For this review, take the finished solid that the model builds, in its own axes (mm). Face numbers are marked on the shaded views. Give positions to 0.01 mm unless a question says otherwise; leave off trailing zeros. Write each loop counter-clockwise with the first axis right and the second up, starting at its lowest first coordinate (ties: lowest second). Pieces come first, ordered by that corner, then holes. Notation, with made-up numbers: M 17.25,-8 L 54.25,-8 A13 ccw 54.25,8 Z; hole C 1,-13.5 d2. An arc over 180 degrees is marked long. Answer as a JSON object with one key per item and string values. Group by question number.
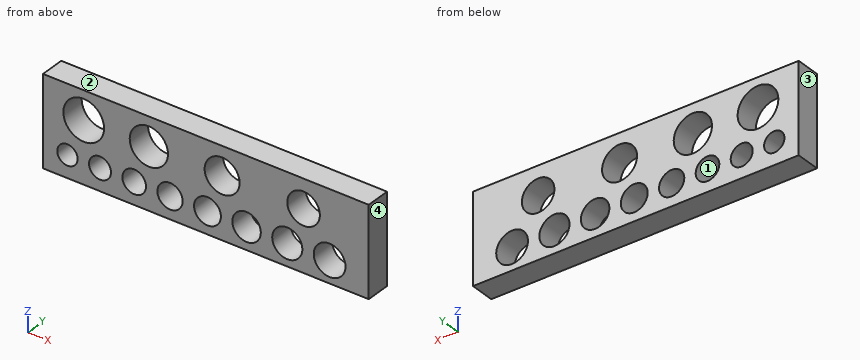
```python
from build123d import *

# Parameters (mm, degrees)
SKETCH1_W           = 40
SKETCH1_H           = 11
BOSS_EXTRUDE1_DEPTH = 3
SKETCH2_R           = 1.25
SKETCH2_R_2         = 1.35
SKETCH2_R_3         = 1.45
SKETCH2_R_4         = 1.55
SKETCH2_R_5         = 1.65
SKETCH2_R_6         = 1.75
SKETCH2_R_7         = 1.85
SKETCH2_R_8         = 1.95
SKETCH2_R_9         = 2.15
SKETCH2_R_10        = 2
SKETCH2_R_11        = 2.5
SKETCH2_R_12        = 2.35
CUT_EXTRUDE1_DEPTH  = 21.958291915


with BuildPart() as part:
    # Sketch1 → Boss-Extrude1 (new body)
    with BuildSketch(Plane(origin=(0, 0, 0), x_dir=(1, 0, 0), z_dir=(0, 1, 0))):
        Rectangle(SKETCH1_W, SKETCH1_H)
    extrude(amount=BOSS_EXTRUDE1_DEPTH)

    # Sketch2 → Cut-Extrude1 (cut, through all)
    with BuildSketch(Plane(origin=(0, 3, 0), x_dir=(1, 0, 0), z_dir=(0, 1, 0))):
        with Locations(Location((-17, 2.8, 0), (0, 0, 270))):
            Circle(SKETCH2_R)
        with Locations(Location((-13, 2.8, 0), (0, 0, 270))):
            Circle(SKETCH2_R_2)
        with Locations(Location((-8.8, 2.8, 0), (0, 0, 270))):
            Circle(SKETCH2_R_3)
        with Locations(Location((-4.4, 2.8, 0), (0, 0, 270))):
            Circle(SKETCH2_R_4)
        with Locations(Location((0.2, 2.8, 0), (0, 0, 270))):
            Circle(SKETCH2_R_5)
        with Locations(Location((5, 2.8, 0), (0, 0, 270))):
            Circle(SKETCH2_R_6)
        with Locations(Location((10, 2.8, 0), (0, 0, 270))):
            Circle(SKETCH2_R_7)
        with Locations(Location((15.2, 2.8, 0), (0, 0, 270))):
            Circle(SKETCH2_R_8)
        with Locations(Location((2, -2, 0), (0, 0, 270))):
            Circle(SKETCH2_R_9)
        with Locations(Location((12, -2, 0), (0, 0, 270))):
            Circle(SKETCH2_R_10)
        with Locations(Location((-15, -2, 0), (0, 0, 270))):
            Circle(SKETCH2_R_11)
        with Locations(Location((-7, -2, 0), (0, 0, 270))):
            Circle(SKETCH2_R_12)
    extrude(amount=-CUT_EXTRUDE1_DEPTH, mode=Mode.SUBTRACT)


solid = part.part
```
Item 1: Consider section B-B (x = 5). Give the boundary of the cut face in (y, z).
Item 2: Consider section A-A (z = 2). Give the boundary of the cut face in (x, y), plus the area to 3 significant figures.
Item 3: Insertion check: P1, Ø4.5, axis at x = 12, z = 2, coming from the -Y side. The pin has a flat end and moves straight along its axis. Give the tip position at first contact, or say it passes through.
Item 4: Draft analysis for pull direction X (two halves, no side actions). For the marked faces 1, 2, 3 and 4, state which applies: released by +X, released by -X, zero draft, split by the parting line, or undercut.
Item 5: Consider section C-C (y = 2.4). State how many separate pieces and enclosed holes the cut face has, plus the area to 3 significant figures.
Item 6: To check wall thickness, follow probe 1 along X at (y, z) = (1.05, 2); probe 2 along X at (y, z) = (0.65, 1); probe 3 along Z at (x, y) = (14.5, 2.3). State the ranges of each line that lie inside material, in increasing order.
Item 7: Consider section D-D (x = -8.8). Give the boundary of the cut face in (y, z), plus the area to 3 significant figures.
Result set:
{
 "1": {"outline": "M 0,-5.5 L 3,-5.5 L 3,-4.55 L 0,-4.55 Z; M 0,-1.05 L 3,-1.05 L 3,5.5 L 0,5.5 Z"},
 "2": {"outline": "M -20,0 L -17.5,0 L -17.5,3 L -20,3 Z; M -12.5,0 L -9.35,0 L -9.35,3 L -12.5,3 Z; M -4.65,0 L -0.15,0 L -0.15,3 L -4.65,3 Z; M 4.15,0 L 10,0 L 10,3 L 4.15,3 Z; M 14,0 L 20,0 L 20,3 L 14,3 Z", "area": "66.0 mm^2"},
 "3": {"P1": "stops at y = 0"},
 "4": {"face 1": "undercut", "face 2": "zero draft", "face 3": "released by -X", "face 4": "released by +X"},
 "5": {"separate pieces": "1", "enclosed holes": "12", "area": "310 mm^2"},
 "6": {"probe 1": "x = -20 to -17.5, -12.5 to -9.35, -4.65 to -0.15, 4.15 to 10, 14 to 20", "probe 2": "x = -20 to -17.29, -12.71 to -9.13, -4.87 to 0.1, 3.9 to 10.27, 13.73 to 20", "probe 3": "z = -5.5 to -4.62, -0.98 to 5.5"},
 "7": {"outline": "M 0,-5.5 L 3,-5.5 L 3,-4.25 L 0,-4.25 Z; M 0,-1.35 L 3,-1.35 L 3,0.49 L 0,0.49 Z; M 0,3.51 L 3,3.51 L 3,5.5 L 0,5.5 Z", "area": "15.2 mm^2"}
}
